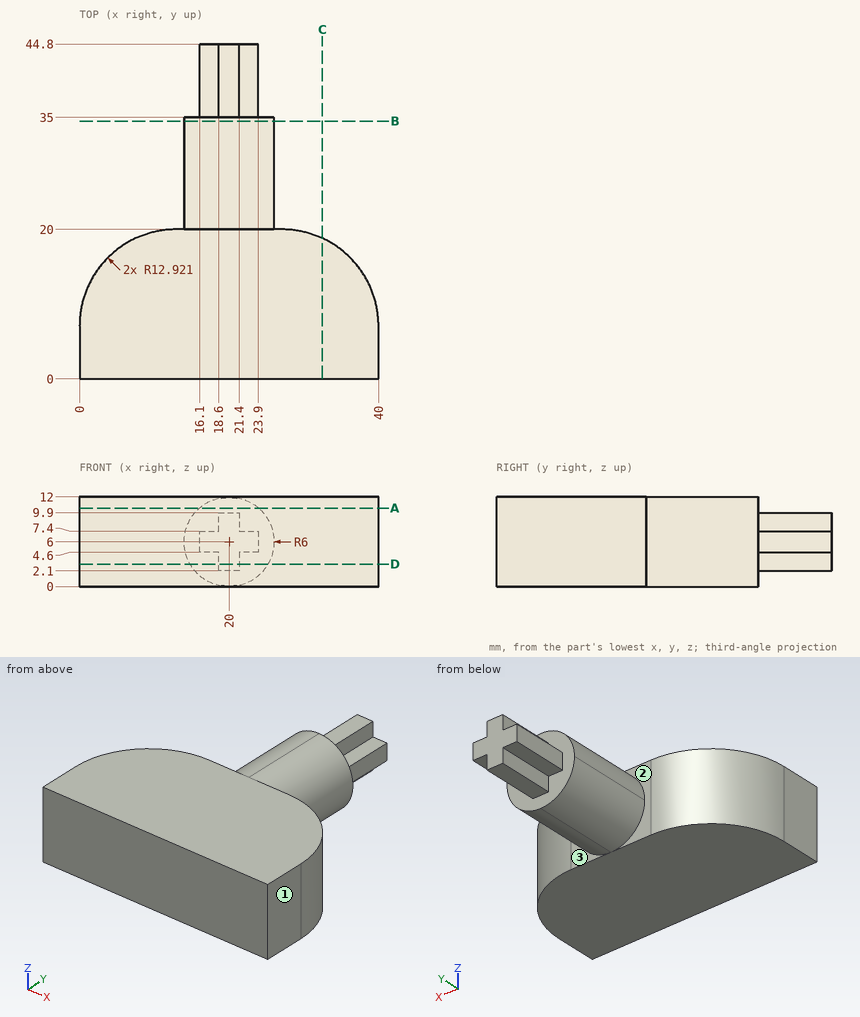
Input: dimensioned drawing with shaded views. Units: mm. Origin: part minimum x, y, z. A direction names the side the tool comes from. Give positions to 0.01 mm unless a question says otherwise; leave off trailing zeros. Loops run counter-clockwise (first coordinate to the right, second up) from the corner with the lowest first, then second, coordinate; pieces in that order, holes last. Notation, with made-up numbers: M 26.5,-11.75 L 49.5,-11.75 A17 cw 49.5,16.25 Z; hole C 82.25,18.25 d4. An arc over 180 degrees is marked long. Put each result on its own line as item: value.
1) Cut plane C-C, the plane x = 32.5. Return the cut outline in (y, z), plus the area to 3 significant figures.
Computed values:
outline: M 0,0 L 18.81,0 L 18.81,12 L 0,12 Z
area: 226 mm^2
2) Cut plane A-A, the plane z = 10.5. Return the cut outline in (x, y).
Computed values:
outline: M 0,0 L 40,0 L 40,7.08 A12.92 ccw 27.08,20 L 23.97,20 L 23.97,35 L 16.03,35 L 16.03,20 L 12.92,20 A12.92 ccw 0,7.08 Z
3) Material intervals for L1, parallel to Y at x = 16.5, z = 3; L2, parallel to Y at x = 15.5, z = 1; L3, parallel to X at y = 42.5, z = 4.5, sorted ascending. Write a range as from..to.
Computed values:
L1: y = 0..35
L2: y = 0..20
L3: x = 18.6..21.4
4) First-contact query: P1, Ø1.5, axis at x = 25, z = 6, coming from the +Y side; P2, Ø3, axis at x = 18, y = 40.5, coming from the +Z side; P3, Ø3, axis at x = 33.5, z = 10, coming from the +Y side; P4, Ø5, axis at x = 33.5, y = 23.5, coming from the +Z side. Flat tips, straight axial feed; report the tip coordinate or a pass-through.
Computed values:
P1: stops at y = 35
P2: stops at z = 9.9
P3: stops at y = 19.03
P4: passes through
5) Cut plane B-B, the plane y = 34.5. Return the cut outline in (x, z), plus the area to 3 significant figures.
Computed values:
outline: M 14,6 A6 ccw 20,0 A6 ccw 20,12 A6 ccw Z
area: 113 mm^2
6) Cut plane D-D, the plane z = 3. Return the cut outline in (x, y).
Computed values:
outline: M 0,0 L 40,0 L 40,7.08 A12.92 ccw 27.08,20 L 25.2,20 L 25.2,35 L 21.4,35 L 21.4,44.8 L 18.6,44.8 L 18.6,35 L 14.8,35 L 14.8,20 L 12.92,20 A12.92 ccw 0,7.08 Z
7) Reachability of the marked faces 1, 2 and 3 from +Z, -Z, +X, -X, +Y, -Y: full face, straight path, thin tool, end or side. Return the list, or none.
Computed values:
face 1: +Z, -Z, +X, +Y, -Y
face 2: -X, +Y
face 3: +X, +Y
